Model file for the job. Use its own axes, mm. Face numbers are marked on the shaded views. Coordinates: 2 decimals unless noted, no trailing zeros. Write each loop counter-clockwise with the first axis right and the second up, starting at its lowest first coordinate (ties: lowest second). Pieces come first, ordered by that corner, then holes. Notation, with made-up numbers: M 66,60 L 120,60 A12 ccw 120,81 Z; hole C 71,49 d10. An arc over 180 degrees is marked long. Put each result on its own line as item: value. Start each with the question number.
Q1. Cut at A-A (z = 22.5). Write the cut outline in (x, y).
Q2. Pull direction Y, two halves, no side cores. Call the marked faces 1, 2 and 3: pulls with the +Y half, pulls with the -Y half, needs draft (parallel to the pull), parting line crosses it, or undercut.
Q3. Drill centre lines: line 1 along Z through (x, y) = (-5, 0); line 2 along Z through (x, y) = (-6.25, 3.5); line 3 along Y through (x, z) = (-7.5, -2.5). Where is each one in solid material? Low to high.
Q4. Cut at C-C (x = -2.25). Write the cut outline in (y, z), then the cut area to 3 significant figures.
Q5. Drop a flat-ended pin along its axis: pin 1 (16 mm diameter, centred on y = 22.5, z = 0, fed in from -X). Give the stop position or say it passes through.
```python
from build123d import *

# Parameters (mm, degrees)
F0_R     = 5
F1_DEPTH = 10


with BuildPart() as f1:
    # F0 (on Right) → F1 (new body)
    with BuildSketch(Plane.YZ):
        Polygon((22.5, 37.9), (0, 37.9), (-15.4, 37.9), (-15.4, 15), (-15.4, 7.5), (-15.4, -15.4), (0, -15.4), (22.5, -15.4), (37.9, -15.4), (37.9, 0), (37.9, 22.5), (37.9, 37.9), align=None)
        Circle(F0_R, mode=Mode.SUBTRACT)
        with Locations((22.5, 0)):
            Circle(F0_R, mode=Mode.SUBTRACT)
        with Locations((0, 22.5)):
            Circle(F0_R, mode=Mode.SUBTRACT)
        with Locations((22.5, 22.5)):
            Circle(F0_R, mode=Mode.SUBTRACT)
    extrude(amount=-F1_DEPTH)


solid = f1.part
```
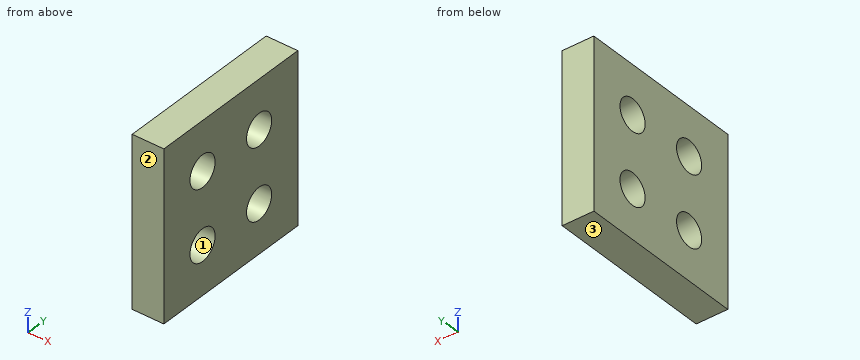
Computed values:
1. outline: M -10,-15.4 L 0,-15.4 L 0,-5 L -10,-5 Z; M -10,5 L 0,5 L 0,17.5 L -10,17.5 Z; M -10,27.5 L 0,27.5 L 0,37.9 L -10,37.9 Z
2. face 1: undercut
2. face 2: pulls with the -Y half
2. face 3: needs draft
3. line 1: -15.4 to -5, 5 to 17.5, 27.5 to 37.9
3. line 2: -15.4 to -3.57, 3.57 to 18.93, 26.07 to 37.9
3. line 3: -15.4 to -4.33, 4.33 to 18.17, 26.83 to 37.9
4. outline: M -15.4,-15.4 L 37.9,-15.4 L 37.9,37.9 L -15.4,37.9 Z; hole C 0,0 d10; hole C 0,22.5 d10; hole C 22.5,0 d10; hole C 22.5,22.5 d10
4. area: 2,530 mm2
5. pin 1: x = -10
